Work out the finished part from the listing and answer in its coordinate system (mm). Round coordinates to 2 decimals unless told otherwise and drop trailing zeros. Write each loop counter-clockwise with the first axis right and the second up, starting at its lowest first coordinate (ties: lowest second). Pieces come first, ordered by that corner, then holes. Notation, with made-up numbers: (-36.5, 6.25) - (3.5, 6.25) arc R21 cw to (3.5, 21.25) - close; hole circle Ø5 at (47.25, 64.5). An arc over 180 degrees is marked (long way). Answer as a JSON object with one key per item and string values.
```python
from build123d import *

# Parameters (mm, degrees)
F0_W     = 68.58
F0_H     = 49.7
F1_DEPTH = 3


with BuildPart() as f1:
    # F0 (on Top) → F1 (new body)
    with BuildSketch(Plane.XY):
        with BuildLine():
            ThreePointArc((-59, 22.85), (-57.5857864376, 23.4357864376), (-57, 24.85))
            Line((-57, 24.85), (-59, 24.85))
            Line((-59, 24.85), (-59, 22.85))
        make_face()
        with BuildLine():
            Line((-59, 24.85), (-57, 24.85))
            ThreePointArc((-57, 24.85), (-60.4142135624, 26.2642135624), (-59, 22.85))
            Line((-59, 22.85), (-59, 24.85))
        make_face()
        with BuildLine():
            Line((-34.29, 24.85), (-57, 24.85))
            ThreePointArc((-57, 24.85), (-57.5857864376, 23.4357864376), (-59, 22.85))
            Line((-59, 22.85), (-59, -22.85))
            ThreePointArc((-59, -22.85), (-57.5857864376, -23.4357864376), (-57, -24.85))
            Line((-57, -24.85), (-34.29, -24.85))
            Line((-34.29, -24.85), (-34.29, 24.85))
        make_face()
        with BuildLine():
            Line((-34.29, 24.94), (-34.29, 24.85))
            Line((-34.29, 24.85), (34.29, 24.85))
            Line((34.29, 24.85), (34.29, 24.94))
            ThreePointArc((34.29, 24.94), (32.8757864376, 25.5257864376), (32.29, 26.94))
            Line((32.29, 26.94), (-32.29, 26.94))
            ThreePointArc((-32.29, 26.94), (-32.8757864376, 25.5257864376), (-34.29, 24.94))
        make_face()
        Rectangle(F0_W, F0_H)
        with BuildLine():
            Line((57, 24.85), (34.29, 24.85))
            Line((34.29, 24.85), (34.29, -24.85))
            Line((34.29, -24.85), (57, -24.85))
            ThreePointArc((57, -24.85), (57.5857864376, -23.4357864376), (59, -22.85))
            Line((59, -22.85), (59, 22.85))
            ThreePointArc((59, 22.85), (57.5857864376, 23.4357864376), (57, 24.85))
        make_face()
        with BuildLine():
            ThreePointArc((-32.29, 26.94), (-35.7042135624, 28.3542135624), (-34.29, 24.94))
            Line((-34.29, 24.94), (-34.29, 26.94))
            Line((-34.29, 26.94), (-32.29, 26.94))
        make_face()
        with BuildLine():
            Line((-34.29, 26.94), (-34.29, 24.94))
            ThreePointArc((-34.29, 24.94), (-32.8757864376, 25.5257864376), (-32.29, 26.94))
            Line((-32.29, 26.94), (-34.29, 26.94))
        make_face()
        with BuildLine():
            Line((34.29, -24.85), (-34.29, -24.85))
            Line((-34.29, -24.85), (-34.29, -24.94))
            ThreePointArc((-34.29, -24.94), (-32.8757864376, -25.5257864376), (-32.29, -26.94))
            Line((-32.29, -26.94), (32.29, -26.94))
            ThreePointArc((32.29, -26.94), (32.8757864376, -25.5257864376), (34.29, -24.94))
            Line((34.29, -24.94), (34.29, -24.85))
        make_face()
        with BuildLine():
            ThreePointArc((-57, -24.85), (-57.5857864376, -23.4357864376), (-59, -22.85))
            Line((-59, -22.85), (-59, -24.85))
            Line((-59, -24.85), (-57, -24.85))
        make_face()
        with BuildLine():
            Line((-59, -24.85), (-59, -22.85))
            ThreePointArc((-59, -22.85), (-60.4142135624, -26.2642135624), (-57, -24.85))
            Line((-57, -24.85), (-59, -24.85))
        make_face()
        with BuildLine():
            ThreePointArc((61, 24.85), (59, 26.85), (57, 24.85))
            Line((57, 24.85), (59, 24.85))
            Line((59, 24.85), (59, 22.85))
            ThreePointArc((59, 22.85), (60.4142135624, 23.4357864376), (61, 24.85))
        make_face()
        with BuildLine():
            Line((59, 24.85), (57, 24.85))
            ThreePointArc((57, 24.85), (57.5857864376, 23.4357864376), (59, 22.85))
            Line((59, 22.85), (59, 24.85))
        make_face()
        with BuildLine():
            ThreePointArc((32.29, 26.94), (32.8757864376, 25.5257864376), (34.29, 24.94))
            Line((34.29, 24.94), (34.29, 26.94))
            Line((34.29, 26.94), (32.29, 26.94))
        make_face()
        with BuildLine():
            Line((34.29, 26.94), (34.29, 24.94))
            ThreePointArc((34.29, 24.94), (35.7042135624, 25.5257864376), (36.29, 26.94))
            ThreePointArc((36.29, 26.94), (34.29, 28.94), (32.29, 26.94))
            Line((32.29, 26.94), (34.29, 26.94))
        make_face()
        with BuildLine():
            ThreePointArc((-32.29, -26.94), (-32.8757864376, -25.5257864376), (-34.29, -24.94))
            Line((-34.29, -24.94), (-34.29, -26.94))
            Line((-34.29, -26.94), (-32.29, -26.94))
        make_face()
        with BuildLine():
            Line((-34.29, -26.94), (-34.29, -24.94))
            ThreePointArc((-34.29, -24.94), (-35.7042135624, -28.3542135624), (-32.29, -26.94))
            Line((-32.29, -26.94), (-34.29, -26.94))
        make_face()
        with BuildLine():
            ThreePointArc((59, -22.85), (57.5857864376, -23.4357864376), (57, -24.85))
            Line((57, -24.85), (59, -24.85))
            Line((59, -24.85), (59, -22.85))
        make_face()
        with BuildLine():
            Line((59, -24.85), (57, -24.85))
            ThreePointArc((57, -24.85), (59, -26.85), (61, -24.85))
            ThreePointArc((61, -24.85), (60.4142135624, -23.4357864376), (59, -22.85))
            Line((59, -22.85), (59, -24.85))
        make_face()
        with BuildLine():
            ThreePointArc((36.29, -26.94), (35.7042135624, -25.5257864376), (34.29, -24.94))
            Line((34.29, -24.94), (34.29, -26.94))
            Line((34.29, -26.94), (32.29, -26.94))
            ThreePointArc((32.29, -26.94), (34.29, -28.94), (36.29, -26.94))
        make_face()
        with BuildLine():
            Line((34.29, -26.94), (34.29, -24.94))
            ThreePointArc((34.29, -24.94), (32.8757864376, -25.5257864376), (32.29, -26.94))
            Line((32.29, -26.94), (34.29, -26.94))
        make_face()
    extrude(amount=F1_DEPTH)


solid = f1.part
```
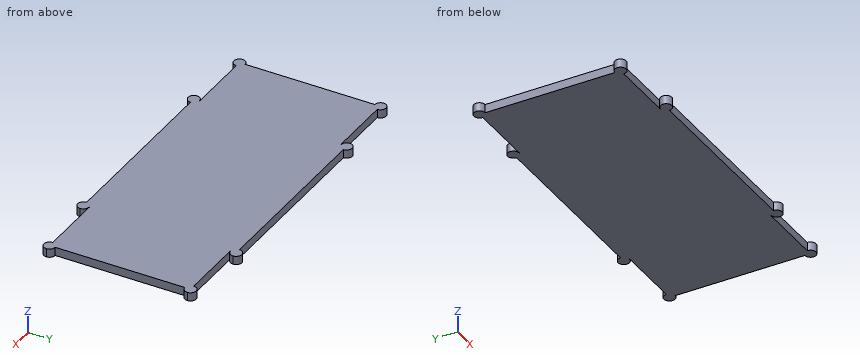
Item 1: A cutting plane is placed at A-A (z = 1.15). Write down the section's boundary in (x, y).
Results found:
{"outline": "(-59, -22.85) arc R2 ccw (long way) to (-57, -24.85) - (-34.29, -24.85) - (-34.29, -24.94) arc R2 ccw (long way) to (-32.29, -26.94) - (32.29, -26.94) arc R2 ccw (long way) to (34.29, -24.94) - (34.29, -24.85) - (57, -24.85) arc R2 ccw (long way) to (59, -22.85) - (59, 22.85) arc R2 ccw (long way) to (57, 24.85) - (34.29, 24.85) - (34.29, 24.94) arc R2 ccw (long way) to (32.29, 26.94) - (-32.29, 26.94) arc R2 ccw (long way) to (-34.29, 24.94) - (-34.29, 24.85) - (-57, 24.85) arc R2 ccw (long way) to (-59, 22.85) - close"}
Item 2: A cutting plane is placed at B-B (y = -14). Write down the section's boundary in (x, z).
Results found:
{"outline": "(-59, 0) - (59, 0) - (59, 3) - (-59, 3) - close"}
Item 3: Each of these flat-tipped pins is pushed along its axis until it touches: P1, Ø0.9, axis at x = 50, z = 1.5, coming from the +Y side; P2, Ø0.9, axis at x = -45.5, z = 2, coming from the -Y side; P3, Ø1.5, axis at y = 9, z = 1.5, coming from the -X side. Where does it stop, or does it pass through?
Results found:
{"P1": "y = 24.85", "P2": "y = -24.85", "P3": "x = -59"}
Item 4: A cutting plane is placed at C-C (x = -9.5). Write down the section's boundary in (y, z), and give its area (3 significant figures).
Results found:
{"outline": "(-26.94, 0) - (26.94, 0) - (26.94, 3) - (-26.94, 3) - close", "area": "162 mm²"}
Item 5: Consider line 1 along Y through (x, z) = (35, 0.7); line 2 along X through (y, z) = (-12.5, 2.2); line 3 along Y through (x, z) = (35.5, 1.2). Determine where each line is inside the solid, lowest interval first.
Results found:
{"line 1": "-28.81 to -25.07, -24.85 to 24.85, 25.07 to 28.81", "line 2": "-59 to 59", "line 3": "-28.53 to -25.35, -24.85 to 24.85, 25.35 to 28.53"}
